```python
from build123d import *

# Parameters (mm, degrees)
SKETCH1_W                                           = 7.62
SKETCH1_H                                           = 26.854156748
BOSS_EXTRUDE1_DEPTH                                 = 2.54
SKETCH2_W                                           = 7.62
SKETCH2_H                                           = 2.54
BOSS_EXTRUDE2_DEPTH                                 = 7.62
CBORE_FOR_4_BINDING_HEAD_MACHINE_SCREW3_D           = 3.175
CBORE_FOR_4_BINDING_HEAD_MACHINE_SCREW3_DEPTH       = 2.54
CBORE_FOR_4_BINDING_HEAD_MACHINE_SCREW3_CBORE_D     = 6.35
CBORE_FOR_4_BINDING_HEAD_MACHINE_SCREW3_CBORE_DEPTH = 2.032
CBORE_FOR_4_BINDING_HEAD_MACHINE_SCREW4_D           = 3.175
CBORE_FOR_4_BINDING_HEAD_MACHINE_SCREW4_DEPTH       = 2.54
CBORE_FOR_4_BINDING_HEAD_MACHINE_SCREW4_CBORE_D     = 6.35
CBORE_FOR_4_BINDING_HEAD_MACHINE_SCREW4_CBORE_DEPTH = 2.032


with BuildPart() as part:
    # Sketch1 → Boss-Extrude1 (new body)
    with BuildSketch(Plane(origin=(-67.768700971, 0, -67.768700971), x_dir=(0.707106781, 0, -0.707106781), z_dir=(0.707106781, 0, 0.707106781))):
        with Locations((-15.829754227, 13.427078374)):
            Rectangle(SKETCH1_W, SKETCH1_H)
        with BuildLine():
            Line((-14.242254227, 22.409156748), (-14.242254227, 4.445))
            ThreePointArc((-14.242254227, 4.445), (-15.829754227, 2.8575), (-17.417254227, 4.445))
            Line((-17.417254227, 4.445), (-17.417254227, 22.409156748))
            ThreePointArc((-17.417254227, 22.409156748), (-15.829754227, 23.996656748), (-14.242254227, 22.409156748))
        make_face(mode=Mode.SUBTRACT)
    extrude(amount=-BOSS_EXTRUDE1_DEPTH)

    # Sketch2 → Boss-Extrude2 (add)
    with BuildSketch(Plane(origin=(-69.564752195, 0, -69.564752195), x_dir=(-0.707106781, 0, 0.707106781), z_dir=(-0.707106781, 0, -0.707106781))):
        with Locations((15.829754227, 25.584156748)):
            Rectangle(SKETCH2_W, SKETCH2_H)
        with Locations((15.829754227, 1.27)):
            Rectangle(SKETCH2_W, SKETCH2_H)
    extrude(amount=BOSS_EXTRUDE2_DEPTH)

    # CBORE for #4 Binding Head Machine Screw3
    with Locations(Plane(origin=(0, 2.54, 0), x_dir=(1, 0, 0), z_dir=(0, 1, 0))):
        with Locations((-83.45215559, 61.065502473)):
            CounterBoreHole(CBORE_FOR_4_BINDING_HEAD_MACHINE_SCREW3_D / 2, CBORE_FOR_4_BINDING_HEAD_MACHINE_SCREW3_CBORE_D / 2, CBORE_FOR_4_BINDING_HEAD_MACHINE_SCREW3_CBORE_DEPTH, depth=CBORE_FOR_4_BINDING_HEAD_MACHINE_SCREW3_DEPTH)

    # CBORE for #4 Binding Head Machine Screw4
    with Locations(Plane(origin=(0, 24.314156748, 0), x_dir=(-1, 0, 0), z_dir=(0, -1, 0))):
        with Locations((83.45215559, 61.065502473)):
            CounterBoreHole(CBORE_FOR_4_BINDING_HEAD_MACHINE_SCREW4_D / 2, CBORE_FOR_4_BINDING_HEAD_MACHINE_SCREW4_CBORE_D / 2, CBORE_FOR_4_BINDING_HEAD_MACHINE_SCREW4_CBORE_DEPTH, depth=CBORE_FOR_4_BINDING_HEAD_MACHINE_SCREW4_DEPTH)


solid = part.part
```
Can you work these out from the model? Positions are in its coordinate system, mm. A direction names the side the tool comes from. Round coordinates to 2 decimals unless told otherwise and drop trailing zeros. Order: outer loops, then holes, each group sorted by start corner. A loop starts at its lowest first (then second) coordinate and runs counter-clockwise, first axis right, second up. Notation, with made-up numbers: (68.5, 20) -> (89.5, 20) arc R28 ccw to (89.5, 44) -> close; hole circle Ø8 at (-3.5, -10.5). An arc over 180 degrees is marked (long way). Return JSON: item names as keys, results as strings. Group by question number.
1. If we section it at D-D, the plane z = -60: Write out the boundary of the cut face in (x, y), then the cut area to 3 significant figures.
2. If we section it at C-C, the plane z = -65.25: Write out the boundary of the cut face in (x, y).
3. If we section it at A-A, the plane y = 9.75: Write out the boundary of the cut face in (x, z).
4. We'd pull the mould along X, two halves only. Please class faces 1 (the face through (-79.872, 23.996, -57.436)), 2 (the face through (-81.99, 13.58, -57.14)), 3 (the face through (-83, 0, -59)), 4 (the face through (-77, 13, -60)): released by +X, released by -X, zero draft, split by the parting line, or undercut.
5. Will these pins go through, and if not, where does the flat tip stop? pin 1 (1.9 mm diameter, centred on x = -82, z = -60.5, fed in from +Y); pin 2 (3 mm diameter, centred on y = 9.5, z = -58, fed in from +X); pin 3 (2 mm diameter, centred on x = -84.5, y = 7, fed in from -Z).
6. Which directions (+Z, -Z, +X, -X, +Y, -Y) give clear straight access to the entire face, cutting with the end or side of a thin tool? Please do faces 5 (the face through (-79.82, 2.86, -57.49)), 6 (the face through (-78.72, 13.55, -58.58)), 7 (the face through (-81.986, 26.604, -60.457)), 8 (the face through (-85.8, 2.54, -58.7)).
7. I need wall thicknesses on line 1 (Y direction, x = -83.5, z = -63.5); line 2 (X direction, y = 24.5, z = -62.25); line 3 (Z direction, x = -82, y = 10). Which ranges of each line are inside material? Lowest first, please. Write a range as [from, to].
Output values:
{
 "1": {"outline": "(-87.77, 0) -> (-84.63, 0) -> (-84.63, 0.51) -> (-86.44, 0.51) -> (-86.44, 2.54) -> (-87.77, 2.54) -> close; (-87.77, 24.31) -> (-86.44, 24.31) -> (-86.44, 26.35) -> (-84.63, 26.35) -> (-84.63, 26.85) -> (-87.77, 26.85) -> close; (-82.28, 0) -> (-77, 0) -> (-77, 26.85) -> (-82.28, 26.85) -> (-82.28, 26.35) -> (-80.46, 26.35) -> (-80.46, 24.31) -> (-79.13, 24.31) -> (-79.13, 2.54) -> (-80.46, 2.54) -> (-80.46, 0.51) -> (-82.28, 0.51) -> close", "area": "74.4 mm²"},
 "2": {"outline": "(-84.66, 0) -> (-82.25, 0) -> (-82.25, 2.54) -> (-84.66, 2.54) -> close; (-84.66, 24.31) -> (-82.25, 24.31) -> (-82.25, 26.85) -> (-84.66, 26.85) -> close"},
 "3": {"outline": "(-83.45, -55.68) -> (-81.88, -57.25) -> (-80.08, -55.45) -> (-81.66, -53.88) -> close; (-79.64, -59.49) -> (-78.06, -61.07) -> (-76.27, -59.27) -> (-77.84, -57.7) -> close"},
 "4": {"face 1": "undercut", "face 2": "released by -X", "face 3": "zero draft", "face 4": "released by +X"},
 "5": {"pin 1": "y = 26.85", "pin 2": "x = -76.27", "pin 3": "through"},
 "6": {"face 5": "none", "face 6": "+Z, -X", "face 7": "+Y, -Y", "face 8": "-Z, -X"},
 "7": {"line 1": "[0, 0.51], [26.35, 26.85]", "line 2": "[-87.66, -86.4], [-80.51, -79.25]", "line 3": "[-57.13, -54.23]"}
}
